```python
from build123d import *

# Parameters (mm, degrees)
F0_R     = 14
F0_R_2   = 1.1
F1_DEPTH = 8
F2_R     = 2
F3_DEPTH = 8.001
F6_R     = 0.875
F7_DEPTH = 19.125355653


# Not quite as in the source:
# - a pattern or mirror of a feature is missing from the dataset's text; its kind, count and spacing are read off the source's solid


with BuildPart() as f1:
    # F0 (on Front) → F1 (new body)
    with BuildSketch(Plane.XZ):
        Circle(F0_R)
        with Locations((-8.6602540378, -5)):
            Circle(F0_R_2, mode=Mode.SUBTRACT)
        with Locations((8.6602540378, -5)):
            Circle(F0_R_2, mode=Mode.SUBTRACT)
        with Locations((0, 10)):
            Circle(F0_R_2, mode=Mode.SUBTRACT)
    extrude(amount=F1_DEPTH)

    # F2 (on face) → F3 (cut, through all)
    with BuildSketch(Plane.XZ.offset(8)):
        Circle(F2_R)
    extrude(amount=-F3_DEPTH, mode=Mode.SUBTRACT)

    # F6 (on line) → F7 (cut, through all)
    with BuildSketch(Plane(origin=(0, 0, 0), x_dir=(0, 1, 0), z_dir=(0.8660254038, 0, -0.5))):
        with Locations((-4, 0)):
            Circle(F6_R)
    f7 = extrude(amount=-F7_DEPTH, mode=Mode.SUBTRACT)

    # F7_copies: F7 across plane
    add(f7.mirror(Plane(origin=(2e-05, 0, 0), x_dir=(-1e-06, 0, 1), z_dir=(1, 0, 1e-06))), mode=Mode.SUBTRACT)


solid = f1.part
```
Here's how the part is built. I have some questions about the finished solid (model axes, mm). Round coordinates to 2 decimals unless told otherwise and drop trailing zeros. Order: outer loops, then holes, each group sorted by start corner. A loop starts at its lowest first (then second) coordinate and runs counter-clockwise, first axis right, second up. Notation, with made-up numbers: (-29.5, 50) -> (26.5, 50) arc R15 ccw to (26.5, 68) -> close; hole circle Ø1 at (76, 0.25). An arc over 180 degrees is marked (long way). Use a Markdown table: item, result. Add a question column.
(1) For pin 1 Ø5 at (x, z) = (0, 0) entering from +Y; pin 2 Ø1 at (y, z) = (-5.5, 4) entering from +X; pin 3 Ø3 at (y, z) = (-2, 9) entering from -X; pin 4 Ø1.5 at (y, z) = (-6, -3) entering from -X, each with a flat end and sliding along its axis, tell me the tip position at first contact or that it passes through.
(2) Suppose I cut it at C-C, the plane z = -5. Please give me the cut outline in (x, y), and give its area (3 significant figures).
(3) Suppose I cut it at B-B, the plane y = -6.5. Please give me the cut outline in (x, z).
(4) Suppose I cut it at D-D, the plane z = -0.5. Please give me the cut outline in (x, y), and give its area (3 significant figures).
(5) If we mould it in two halves opening along Z, with no side actions, what happens to faces 1 (the face through (12.932, -3.944, -5.362)), 2 (the face through (0, 0, -3)), 3 (the face through (6.636, -3.165, 4.135))? For each: released by +Z, released by -Z, zero draft, split by the parting line, or undercut.
(6) Suppose I cut it at A-A, the plane x = 0. Please give me the cut outline in (y, z), and give its area (3 significant figures).
(7) I need wall thicknesses on line 1 along Z through (x, y) = (0, -5.75); line 2 along Z through (x, y) = (-1, -1.5); line 3 along X through (y, z) = (-4.5, 5). Which ranges of each line are inside material? Lowest first, please.
Verdict:
| question | item | result |
|---|---|---|
| 1 | pin 1 | y = 0 |
| 1 | pin 2 | x = 13.56 |
| 1 | pin 3 | x = -11.82 |
| 1 | pin 4 | x = -13.82 |
| 2 | outline | (-13.08, -8) -> (-9.76, -8) -> (-9.76, 0) -> (-13.08, 0) -> close; (-7.56, -8) -> (7.56, -8) -> (7.56, 0) -> (-7.56, 0) -> close; (9.76, -8) -> (13.08, -8) -> (13.08, 0) -> (9.76, 0) -> close |
| 2 | area | 174 mm2 |
| 3 | outline | circle Ø28 at (0, 0); hole circle Ø2.2 at (-8.66, -5); hole circle Ø4 at (0, 0); hole circle Ø2.2 at (0, 10); hole circle Ø2.2 at (8.66, -5) |
| 4 | outline | (-13.99, -8) -> (-1.94, -8) -> (-1.94, 0) -> (-13.99, 0) -> close; (1.94, -8) -> (13.99, -8) -> (13.99, 0) -> (1.94, 0) -> close |
| 4 | area | 193 mm2 |
| 5 | face 1 | split by the parting line |
| 5 | face 2 | zero draft |
| 5 | face 3 | undercut |
| 6 | outline | (-8, -14) -> (0, -14) -> (0, -2) -> (-8, -2) -> close; (-8, 2) -> (0, 2) -> (0, 8.9) -> (-8, 8.9) -> close; (-8, 11.1) -> (0, 11.1) -> (0, 14) -> (-8, 14) -> close |
| 6 | area | 174 mm2 |
| 7 | line 1 | -14 to -2, 2 to 8.9, 11.1 to 14 |
| 7 | line 2 | -13.96 to -1.73, 1.73 to 9.54, 10.46 to 13.96 |
| 7 | line 3 | -13.08 to -10.1, -7.22 to 7.22, 10.1 to 13.08 |
